Could you check a few things on this model? Use its own coordinates, in mm. A direction names the side the tool comes from. Round coordinates to 2 decimals unless told otherwise and drop trailing zeros. Loops run counter-clockwise (first coordinate to the right, second up) from the corner with the lowest first, then second, coordinate; pieces in that order, holes last. Notation, with made-up numbers: M 60.25,53 L 82.25,53 A18 cw 82.25,83 Z; hole C -24.5,-24 d8. An arc over 180 degrees is marked long. Return JSON: item names as keys, results as strings. Group by question number.
```python
from build123d import *

# Parameters (mm, degrees)
SKETCH1_W              = 70
SKETCH1_H              = 12
SKETCH1_R              = 1.5
SKETCH1_R_2            = 4.125
BOSS_EXTRUDE1_DEPTH    = 3
BOSS_EXTRUDE2_DEPTH    = 12.5
CUT_EXTRUDE1_START     = -22.5
CUT_EXTRUDE1_OUTLINE_W = 5
CUT_EXTRUDE1_OUTLINE_H = 3
CUT_EXTRUDE1_DEPTH     = 35
CUT_EXTRUDE2_START     = -22.5
CUT_EXTRUDE2_DEPTH     = 22.5
CUT_EXTRUDE3_START     = 8
SKETCH2_5_W            = 32.5
SKETCH2_5_H            = 9.897866997
CUT_EXTRUDE3_DEPTH     = 4.5
SKETCH4_W              = 5
SKETCH4_H              = 13
BOSS_EXTRUDE3_DEPTH    = 3


# Read off the part's stored shape, not the designer's step: Cut-Extrude1
with BuildPart() as part:
    # Sketch1 → Boss-Extrude1 (new body)
    # profile 1 of 2: a face of its own
    with BuildSketch(Plane(origin=(0, 0, 0), x_dir=(1, 0, 0), z_dir=(0, 1, 0))):
        Polygon((82.5, 22.5), (-100, 22.5), (-100, -12.5), (82.5, -12.5), (82.5, -1), (12.5, -1), (12.5, 11), (82.5, 11), align=None)
    # profile 2 of 2: a face of its own
    with BuildSketch(Plane(origin=(0, 0, 0), x_dir=(1, 0, 0), z_dir=(0, 1, 0))):
        with Locations((47.5, 5)):
            Rectangle(SKETCH1_W, SKETCH1_H)
        with Locations(Location((20.5, 5, 0), (0, 0, 270))):
            Circle(SKETCH1_R, mode=Mode.SUBTRACT)
        with Locations(Location((47.5, 5, 0), (0, 0, 270))):
            Circle(SKETCH1_R_2, mode=Mode.SUBTRACT)
        with Locations(Location((74.5, 5, 0), (0, 0, 270))):
            Circle(SKETCH1_R, mode=Mode.SUBTRACT)
    extrude(amount=BOSS_EXTRUDE1_DEPTH)

    # Sketch2 → Boss-Extrude2 (add)
    with BuildSketch(Plane.XY):
        with BuildLine():
            Line((-89, 33), (-89, -17))
            ThreePointArc((-89, -17), (-94.5, -22.5), (-100, -17))
            Line((-100, -17), (-100, 33))
            ThreePointArc((-100, 33), (-94.5, 38.5), (-89, 33))
        make_face()
        with BuildLine():
            ThreePointArc((-97, -17), (-94.5, -19.5), (-92, -17))
            Line((-92, -17), (-92, 33))
            ThreePointArc((-92, 33), (-94.5, 35.5), (-97, 33))
            Line((-97, 33), (-97, -17))
        make_face(mode=Mode.SUBTRACT)
    extrude(amount=BOSS_EXTRUDE2_DEPTH)

    # Cut-Extrude1 outline → Cut-Extrude1 (cut)
    with BuildSketch(Plane.XY.offset(CUT_EXTRUDE1_START)):
        with Locations((-94.5, 1.5)):
            Rectangle(CUT_EXTRUDE1_OUTLINE_W, CUT_EXTRUDE1_OUTLINE_H)
    extrude(amount=CUT_EXTRUDE1_DEPTH, mode=Mode.SUBTRACT)

    # Sketch2<3> → Cut-Extrude2 (cut)
    with BuildSketch(Plane.XY.offset(CUT_EXTRUDE2_START)):
        with BuildLine():
            Line((-89, 33), (-89, -17))
            ThreePointArc((-89, -17), (-94.5, -22.5), (-100, -17))
            Line((-100, -17), (-100, 33))
            ThreePointArc((-100, 33), (-94.5, 38.5), (-89, 33))
        make_face()
        with BuildLine():
            ThreePointArc((-97, -17), (-94.5, -19.5), (-92, -17))
            Line((-92, -17), (-92, 33))
            ThreePointArc((-92, 33), (-94.5, 35.5), (-97, 33))
            Line((-97, 33), (-97, -17))
        make_face(mode=Mode.SUBTRACT)
    extrude(amount=CUT_EXTRUDE2_DEPTH, mode=Mode.SUBTRACT)

    # Sketch2<5> → Cut-Extrude3 (cut)
    with BuildSketch(Plane.XY.offset(CUT_EXTRUDE3_START)):
        with Locations((-66.75, 1.550857661)):
            Rectangle(SKETCH2_5_W, SKETCH2_5_H)
    extrude(amount=CUT_EXTRUDE3_DEPTH, mode=Mode.SUBTRACT)

    # Sketch4 → Boss-Extrude3 (add)
    with BuildSketch(Plane.XY.offset(8)):
        with Locations((-80.5, 9.5)):
            Rectangle(SKETCH4_W, SKETCH4_H)
        with Locations((-53, 9.5)):
            Rectangle(SKETCH4_W, SKETCH4_H)
    extrude(amount=-BOSS_EXTRUDE3_DEPTH)


solid = part.part
```
1. We'd pull the mould along Z, two halves only. Please class faces 4 (the face through (-2, 1, -22.5)), 5 (the face through (43.473, 1.479, -5.894)), 6 (the face through (-4, 3, -5)): +Z half, -Z half, draft (parallel to the pull), parting line (faces both ways), or undercut.
2. If we section it at B-B, the plane y = 7.5: Please give me the cut outline in (x, z).
3. If we section it at D-D, the plane y = -2.5: Please give me the cut outline in (x, z), then the cut area to 3 significant figures.
4. I'm going to push flat-ended pins straight in: pin 1 Ø14 at (y, z) = (13, 5.5) entering from +X; pin 2 Ø3.5 at (y, z) = (1.5, -12.5) entering from -X; pin 3 Ø2.5 at (x, z) = (-52, 7) entering from +Y. Where does each tip first touch, or does it pass through?
5. If we section it at A-A, the plane x = -94.5: Please give me the cut outline in (y, z), then the cut area to 3 significant figures.
6. If we section it at C-C, the plane z = 3: Please give me the cut outline in (x, y).
7. On a 3-axis mill with a long thin cutter (end or side, diameter ignored), from which of +Z, -Z, +X, -X, +Y, -Y can I reach the whole of each face in a straight line? I mean faces 1 (the face through (-94.6, -19.5, 6.2)), 2 (the face through (-83, 9, 7)), 3 (the face through (-81, 10, 5)). Say none if no direction works.
8. I need wall thicknesses on probe 1 along X at (y, z) = (1.1, -5) (3 decimals); probe 2 along Y at (x, z) = (27, -16.5); probe 3 along Z at (x, y) = (47, 1). Which ranges of each line are inside material? Lowest first, please.
Geometry results:
{
 "1": {"face 4": "-Z half", "face 5": "undercut", "face 6": "draft"},
 "2": {"outline": "M -100,0 L -97,0 L -97,12.5 L -100,12.5 Z; M -92,0 L -89,0 L -89,12.5 L -92,12.5 Z; M -83,5 L -78,5 L -78,8 L -83,8 Z; M -55.5,5 L -50.5,5 L -50.5,8 L -55.5,8 Z"},
 "3": {"outline": "M -100,0 L -97,0 L -97,12.5 L -100,12.5 Z; M -92,0 L -89,0 L -89,12.5 L -92,12.5 Z", "area": "75.0 mm^2"},
 "4": {"pin 1": "x = -50.5", "pin 2": "x = -89", "pin 3": "y = 16"},
 "5": {"outline": "M -22.5,0 L -19.5,0 L -19.5,12.5 L -22.5,12.5 Z; M 35.5,0 L 38.5,0 L 38.5,12.5 L 35.5,12.5 Z", "area": "75.0 mm^2"},
 "6": {"outline": "M -100,-17 A5.5 ccw -89,-17 L -89,0 L 82.5,0 L 82.5,3 L -89,3 L -89,33 A5.5 ccw -100,33 Z; hole M -97,-17 A2.5 ccw -92,-17 L -92,33 A2.5 ccw -97,33 Z"},
 "7": {"face 1": "+Z, -Z", "face 2": "+Z, -Z, +Y", "face 3": "-Z, +X, +Y"},
 "8": {"probe 1": "-89 to 19, 22 to 43.375, 51.625 to 73, 76 to 82.5", "probe 2": "0 to 3", "probe 3": "-22.5 to -9.09, -0.91 to 12.5"}
}
